Source: three-view drawing plus pictorial views. Frame: mm from the lowest corner of the part. A direction names the side the tool comes from. Give positions to 0.01 mm unless a question says otherwise; leave off trailing zeros. Loops run counter-clockwise (first coordinate to the right, second up) from the corner with the lowest first, then second, coordinate; pieces in that order, holes last.
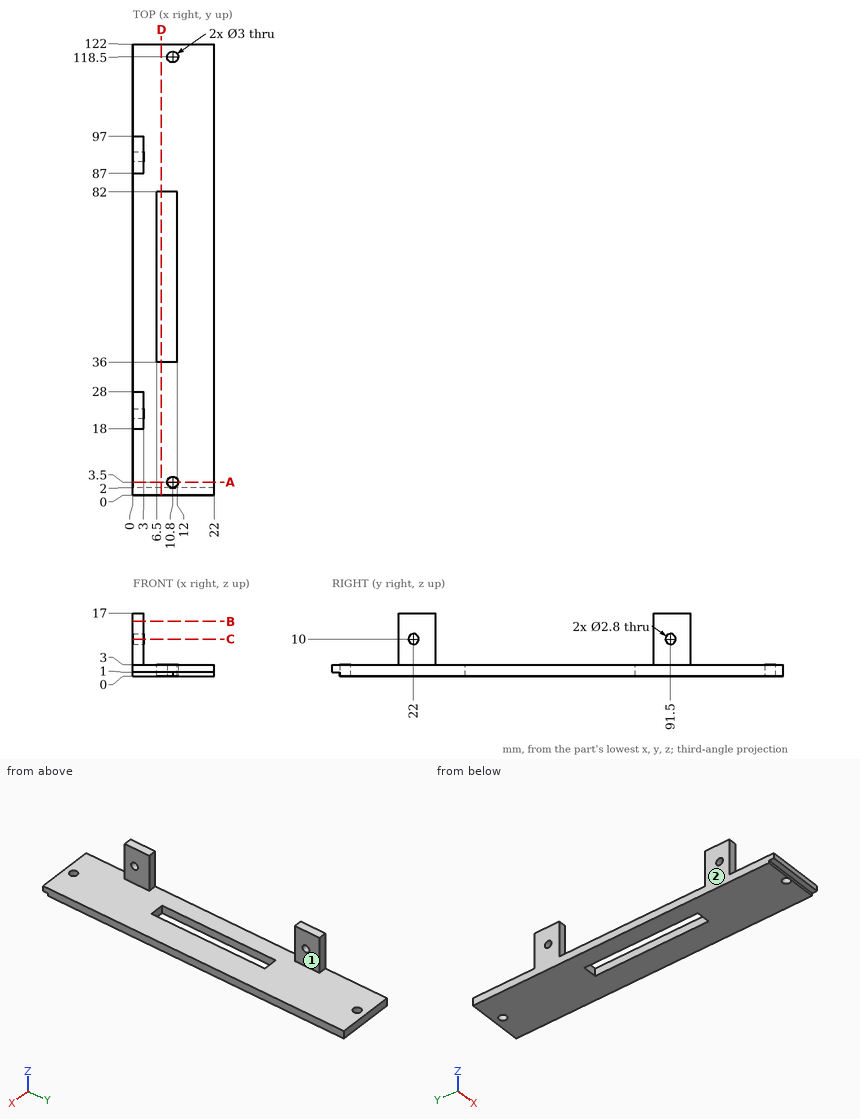
(1) Cut plane D-D (x = 7.75). Return the cut outline in (y, z), and give its area (3 significant figures).
Values follow:
outline: (0, 1) - (2, 1) - (2, 0) - (36, 0) - (36, 3) - (0, 3) - close; (82, 0) - (122, 0) - (122, 3) - (82, 3) - close
area: 226 mm2
(2) Cut plane C-C (z = 10). Return the cut outline in (x, y), and give its area (3 significant figures).
Values follow:
outline: (0, 18) - (3, 18) - (3, 20.6) - (0, 20.6) - close; (0, 23.4) - (3, 23.4) - (3, 28) - (0, 28) - close; (0, 87) - (3, 87) - (3, 90.1) - (0, 90.1) - close; (0, 92.9) - (3, 92.9) - (3, 97) - (0, 97) - close
area: 43.2 mm2
(3) Pin query (flat end, axial travel): pin 1 Ø0.5 at (x, z) = (18.5, 0.5) entering from -Y; pin 2 Ø0.9 at (x, z) = (1, 7) entering from +Y; pin 3 Ø3.5 at (y, z) = (69, 1) entering from -X; pin 4 Ø4 at (x, y) = (16, 25.5) entering from +Z. Return the tip coordinate at first contact, or that it passes through.
Values follow:
pin 1: stops at y = 2
pin 2: stops at y = 97
pin 3: stops at x = 0
pin 4: stops at z = 3
(4) Cut plane B-B (z = 14.75). Return the cut outline in (x, y).
Values follow:
outline: (0, 18) - (3, 18) - (3, 28) - (0, 28) - close; (0, 87) - (3, 87) - (3, 97) - (0, 97) - close
(5) Ray query, probe 1 along Y at (x, z) = (2.3, 10); probe 2 along Z at (x, y) = (1, 91.5); probe 3 along Z at (x, y) = (8, 112.5). Return the intervals inside material, ascending.
Values follow:
probe 1: y = 18 to 20.6, 23.4 to 28, 87 to 90.1, 92.9 to 97
probe 2: z = 0 to 8.6, 11.4 to 17
probe 3: z = 0 to 3
(6) Cut plane A-A (y = 3.5). Return the cut outline in (x, z).
Values follow:
outline: (0, 0) - (9.3, 0) - (9.3, 3) - (0, 3) - close; (12.3, 0) - (22, 0) - (22, 3) - (12.3, 3) - close
(7) Reachability of the marked faces 1 and 2 from +Z, -Z, +X, -X, +Y, -Y: full face, straight path, thin tool, end or side. Return the list, or none.
Values follow:
face 1: +Z, +X, +Y, -Y
face 2: +Z, -Z, -X, +Y, -Y
